```python
from build123d import *

# Parameters (mm, degrees)
CROQUIS1_W            = 15
CROQUIS1_H            = 25
CROQUIS9_W            = 10
CROQUIS9_H            = 10
CROQUIS10_R           = 1.5
CORTAR_EXTRUIR1_DEPTH = 5
CROQUIS11_R           = 2.5
CORTAR_EXTRUIR2_DEPTH = 3


with BuildPart() as part:
    # Croquis1 → Recubrir1 section 0
    with BuildSketch(Plane.XY):
        Rectangle(CROQUIS1_W, CROQUIS1_H)
    # Croquis9 → Recubrir1 section 1
    with BuildSketch(Plane.XY.offset(5)):
        Rectangle(CROQUIS9_W, CROQUIS9_H)
    loft()

    # Croquis10 → Cortar-Extruir1 (cut)
    with BuildSketch(Plane.XY.offset(5)):
        Circle(CROQUIS10_R)
    extrude(amount=-CORTAR_EXTRUIR1_DEPTH, mode=Mode.SUBTRACT)

    # Croquis11 → Cortar-Extruir2 (cut)
    with BuildSketch(Plane(origin=(0, 0, 0), x_dir=(-1, 0, 0), z_dir=(0, 0, -1))):
        Circle(CROQUIS11_R)
    extrude(amount=-CORTAR_EXTRUIR2_DEPTH, mode=Mode.SUBTRACT)


solid = part.part
```
Source: CAD feature listing. Evaluate the final solid. Frame: model axes, mm. A direction names the side the tool comes from. Round coordinates to 2 decimals unless told otherwise and drop trailing zeros. Use a Markdown table: item, result. Add a question column.
1. Reachability of faces 3 (the cylindrical face through (0.54, -2.44, 1.48)), 4 (the cylindrical face through (-1.5, 0.07, 4.01)) from +Z, -Z, +X, -X, +Y, -Y: full face, straight path, thin tool, end or side. Return the list, or none.
2. Contact query for flat-ended pins moving along their axis: P1, Ø2, axis at x = -2.5, y = 9, coming from the +Z side; P2, Ø2.5, axis at x = 0, y = 0, coming from the +Z side. Output: stop coordinate, or through.
3. Mould query, pull axis X, two halves, no side actions, for faces 1 (the flat face through (0, -2, 3)), 2 (the flat face through (-1.3, 1.1, 5)). Classes: pulls with the +X half, pulls with the -X half, needs draft (parallel to the pull), parting line crosses it, or undercut.
4. Line query: line 1 (Z direction, x = 6, y = -5.5); line 2 (Y direction, x = 0, z = 3.7); line 3 (Y direction, x = 0, z = 1.7). Output: solid intervals per line, ascending.
Reported:
| question | item | result |
|---|---|---|
| 1 | face 3 | -Z |
| 1 | face 4 | +Z, -Z |
| 2 | P1 | stops at z = 3 |
| 2 | P2 | passes through |
| 3 | face 1 | undercut |
| 3 | face 2 | needs draft |
| 4 | line 1 | z = 0 to 3 |
| 4 | line 2 | y = -6.95 to -1.5, 1.5 to 6.95 |
| 4 | line 3 | y = -9.95 to -2.5, 2.5 to 9.95 |
